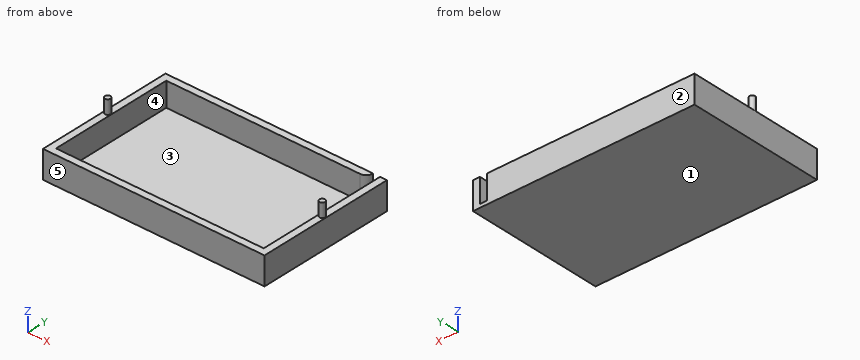
```python
from build123d import *

# Parameters (mm, degrees)
F1_DEPTH = 25.4
F2_DEPTH = 3.175
F3_R     = 2.54
F4_DEPTH = 12.7


with BuildPart() as f1:
    # F0 (on Top) → F1 (new body)
    with BuildSketch(Plane.XY):
        with BuildLine():
            Line((88.9, 63.5), (-101.6, 63.5))
            Line((-101.6, 63.5), (-101.6, -63.5))
            Line((-101.6, -63.5), (101.6, -63.5))
            Line((101.6, -63.5), (101.6, 63.5))
            Line((101.6, 63.5), (95.25, 63.5))
            Line((95.25, 63.5), (95.25, 57.15))
            Line((95.25, 57.15), (95.25, -57.15))
            Line((95.25, -57.15), (-95.25, -57.15))
            Line((-95.25, -57.15), (-95.25, 57.15))
            Line((-95.25, 57.15), (82.55, 57.15))
            ThreePointArc((82.55, 57.15), (87.040128, 59.009872), (88.9, 63.5))
        make_face()
    extrude(amount=F1_DEPTH)

    # F0 (on Top) → F2 (join)
    with BuildSketch(Plane.XY):
        with BuildLine():
            Line((95.25, 63.5), (88.9, 63.5))
            ThreePointArc((88.9, 63.5), (87.040128, 59.009872), (82.55, 57.15))
            Line((82.55, 57.15), (-95.25, 57.15))
            Line((-95.25, 57.15), (-95.25, -57.15))
            Line((-95.25, -57.15), (95.25, -57.15))
            Line((95.25, -57.15), (95.25, 57.15))
            Line((95.25, 57.15), (95.25, 63.5))
        make_face()
    extrude(amount=F2_DEPTH)

    # F3 (on face) → F4 (join)
    with BuildSketch(Plane.XY.offset(25.4)):
        with Locations((-98.425, 0)):
            Circle(F3_R)
        with Locations((98.425, 0)):
            Circle(F3_R)
    extrude(amount=F4_DEPTH)


solid = f1.part
```
The listing builds one solid part. Answer for the finished solid, in the listing's coordinates (mm). Face numbers are marked on the shaded views. A direction names the side the tool comes from. Coordinates: 2 decimals unless noted, no trailing zeros. Write each loop counter-clockwise with the first axis right and the second up, starting at its lowest first coordinate (ties: lowest second). Pieces come first, ordered by that corner, then holes.
Q1. Section D-D, the plane y = 14 is taken. Write down the section's boundary in (x, z) (3 decimals).
Returned:
outline: (-101.6, 0) - (101.6, 0) - (101.6, 25.4) - (95.25, 25.4) - (95.25, 3.175) - (-95.25, 3.175) - (-95.25, 25.4) - (-101.6, 25.4) - close
Q2. Which of the six approach directions +Z, -Z, +X, -X, +Y, -Y give full straight-line access (tool end or side, diameter ignored) to the marked faces 4 and 5?
Returned:
face 4: +Z
face 5: +Z, -Z, +X, -X, -Y
Q3. Find the intervals of material crossed by line 1 along X through (y, z) = (-13, 16); line 2 along Y through (x, z) = (-62.5, 5.5); line 3 along Z through (x, y) = (-17.5, -28.5) (3 decimals), in increasing order.
Returned:
line 1: x = -101.6 to -95.25, 95.25 to 101.6
line 2: y = -63.5 to -57.15, 57.15 to 63.5
line 3: z = 0 to 3.175
Q4. The mould has two halves that part along Y. Classify the marked faces 1, 2 and 3: released by +Y, released by -Y, zero draft, split by the parting line, or undercut.
Returned:
face 1: zero draft
face 2: released by +Y
face 3: undercut
Q5. Section A-A, the plane z = 16.5 is taken. Write down the section's boundary in (x, y), then the cut area to 3 significant figures.
Returned:
outline: (-101.6, -63.5) - (101.6, -63.5) - (101.6, 63.5) - (95.25, 63.5) - (95.25, -57.15) - (-95.25, -57.15) - (-95.25, 57.15) - (82.55, 57.15) arc R6.35 ccw to (88.9, 63.5) - (-101.6, 63.5) - close
area: 3,980 mm2
Q6. Section C-C, the plane x = 43 is taken. Write down the section's boundary in (y, z) (3 decimals).
Returned:
outline: (-63.5, 0) - (63.5, 0) - (63.5, 25.4) - (57.15, 25.4) - (57.15, 3.175) - (-57.15, 3.175) - (-57.15, 25.4) - (-63.5, 25.4) - close
Q7. Section B-B, the plane y = 0 is taken. Write down the section's boundary in (x, z) (3 decimals), then the cut area to 3 significant figures.
Returned:
outline: (-101.6, 0) - (101.6, 0) - (101.6, 25.4) - (100.965, 25.4) - (100.965, 38.1) - (95.885, 38.1) - (95.885, 25.4) - (95.25, 25.4) - (95.25, 3.175) - (-95.25, 3.175) - (-95.25, 25.4) - (-95.885, 25.4) - (-95.885, 38.1) - (-100.965, 38.1) - (-100.965, 25.4) - (-101.6, 25.4) - close
area: 1,060 mm2
